Print and shaded views of the part. All mm, measured from the part's lowest x, y and z. Round coordinates to 2 decimals unless told otherwise and drop trailing zeros. Write each loop counter-clockwise with the first axis right and the second up, starting at its lowest first coordinate (ties: lowest second). Pieces come first, ordered by that corner, then holes. Notation, with made-up numbers: M 32.25,-27 L 54.25,-27 A11 cw 54.25,-13 Z; hole C -9.75,83.5 d7. An arc over 180 degrees is marked long. Write item = value, one per line.
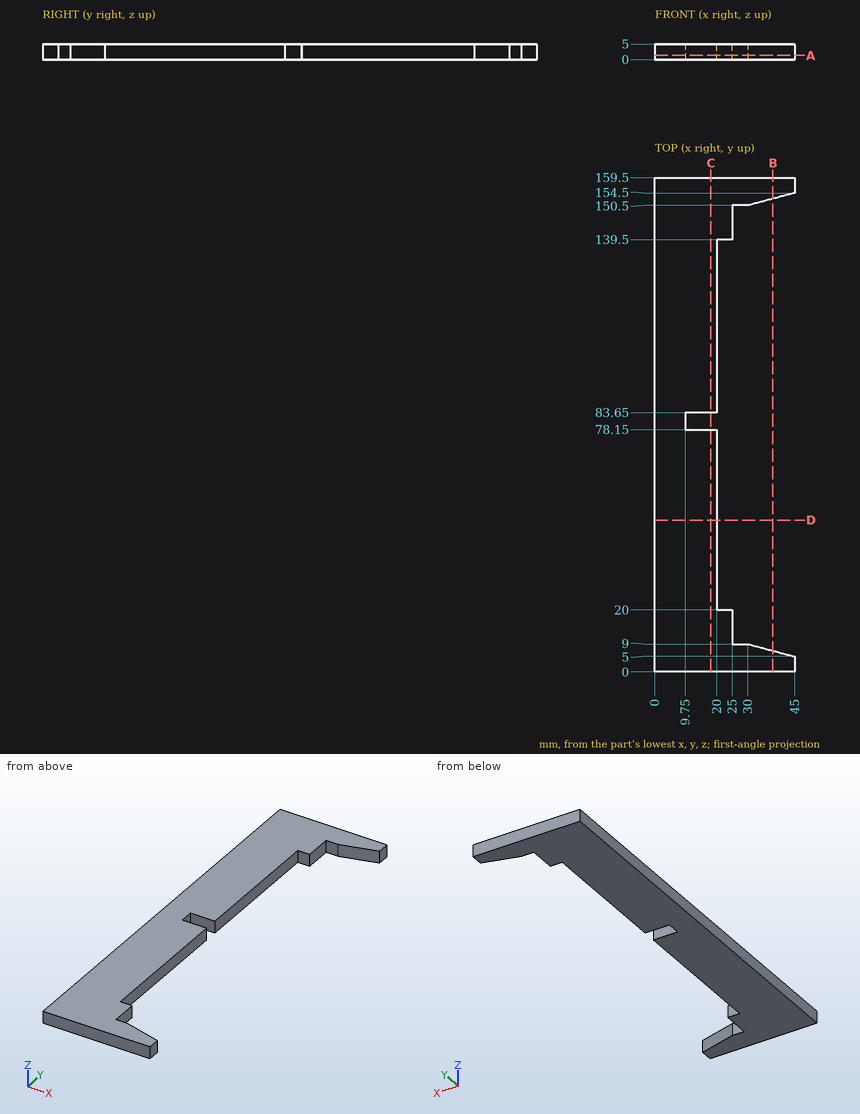
1. Band-saw the part on C-C (x = 18). List the corners of the cut face in (y, z), plus the area to 3 significant figures.
Responses:
outline = M 0,0 L 78.15,0 L 78.15,5 L 0,5 Z; M 83.65,0 L 159.5,0 L 159.5,5 L 83.65,5 Z
area = 770 mm²
2. Band-saw the part on A-A (z = 1.35). List the corners of the cut face in (x, y).
Responses:
outline = M 0,0 L 45,0 L 45,5 L 30,9 L 25,9 L 25,20 L 20,20 L 20,78.15 L 9.75,78.15 L 9.75,83.65 L 20,83.65 L 20,139.5 L 25,139.5 L 25,150.5 L 30,150.5 L 45,154.5 L 45,159.5 L 0,159.5 Z
3. Band-saw the part on B-B (x = 38). List the corners of the cut face in (y, z).
Responses:
outline = M 0,0 L 6.87,0 L 6.87,5 L 0,5 Z; M 152.63,0 L 159.5,0 L 159.5,5 L 152.63,5 Z
4. Band-saw the part on D-D (y = 49). List the corners of the cut face in (x, z), plus the area to 3 significant figures.
Responses:
outline = M 0,0 L 20,0 L 20,5 L 0,5 Z
area = 100 mm²
5. Flat gauge pins, fed straight in: pin 1 (1.5 mm diameter, centred on y = 60, z = 2, fed in from +X); pin 2 (2.5 mm diameter, centred on y = 147, z = 2, fed in from +X). Where does each tip first touch, or does it go through?
Responses:
pin_1 = 20
pin_2 = 25
6. Probe probe 1 along Y at (x, z) = (28.5, 4.65); probe 2 along Y at (x, z) = (11.5, 2.9); probe 3 along X at (y, z) = (138, 3.85). List the from-to ranges inside material, lowest first.
Responses:
probe_1 = 0 to 9, 150.5 to 159.5
probe_2 = 0 to 78.15, 83.65 to 159.5
probe_3 = 0 to 20
